from build123d import *

# Parameters (mm, degrees)
CUT_EXTRUDE1_START     = -5
CUT_EXTRUDE1_OUTLINE_W = 4.8
CUT_EXTRUDE1_OUTLINE_H = 50
CUT_EXTRUDE1_DEPTH     = 5
BOSS_EXTRUDE1_START    = -5
BOSS_EXTRUDE1_DEPTH    = 5
BOSS_EXTRUDE2_START    = -5
BOSS_EXTRUDE2_DEPTH    = 5
CUT_EXTRUDE2_DEPTH     = 10
BOSS_EXTRUDE3_START    = -5
BOSS_EXTRUDE3_DEPTH    = 5
BOSS_EXTRUDE4_START    = -5
BOSS_EXTRUDE4_DEPTH    = 5


with BuildPart() as part:
    # Cut-Extrude1: read off the stored shape, not the designer's step
    # Cut-Extrude1 outline → Cut-Extrude1 (new body)
    with BuildSketch(Plane.ZY.offset(CUT_EXTRUDE1_START)):
        with BuildLine():
            Line((22, -25), (47, -50))
            Line((47, -50), (115, -50))
            Line((115, -50), (115, 50))
            Line((115, 50), (-115, 50))
            Line((-115, 50), (-115, -50))
            Line((-115, -50), (-47, -50))
            Line((-47, -50), (-22, -25))
            Line((-22, -25), (-22, 0))
            ThreePointArc((-22, 0), (-16.382917933, 14.683323874), (-2.4, 21.868699093))
            Line((-2.4, 21.868699093), (-2.4, 25))
            Line((-2.4, 25), (2.4, 25))
            Line((2.4, 25), (2.4, 21.868699093))
            ThreePointArc((2.4, 21.868699093), (16.382917933, 14.683323874), (22, 0))
            Line((22, 0), (22, -25))
        make_face()
        with BuildLine():
            ThreePointArc((-33.2, -22.75), (-30.95, -25), (-33.2, -27.25))
            Line((-33.2, -27.25), (-93.2, -27.25))
            ThreePointArc((-93.2, -27.25), (-95.45, -25), (-93.2, -22.75))
            Line((-93.2, -22.75), (-33.2, -22.75))
        make_face(mode=Mode.SUBTRACT)
        with BuildLine():
            ThreePointArc((33.2, -27.25), (30.95, -25), (33.2, -22.75))
            Line((33.2, -22.75), (93.2, -22.75))
            ThreePointArc((93.2, -22.75), (95.45, -25), (93.2, -27.25))
            Line((93.2, -27.25), (33.2, -27.25))
        make_face(mode=Mode.SUBTRACT)
        with Locations((-100, 0)):
            Rectangle(CUT_EXTRUDE1_OUTLINE_W, CUT_EXTRUDE1_OUTLINE_H, mode=Mode.SUBTRACT)
        with BuildLine():
            ThreePointArc((-58.2, 19.5), (-38.7, 0), (-58.2, -19.5))
            Line((-58.2, -19.5), (-68.2, -19.5))
            ThreePointArc((-68.2, -19.5), (-87.7, 0), (-68.2, 19.5))
            Line((-68.2, 19.5), (-58.2, 19.5))
        make_face(mode=Mode.SUBTRACT)
        with BuildLine():
            ThreePointArc((-33.2, 27.25), (-30.95, 25), (-33.2, 22.75))
            Line((-33.2, 22.75), (-93.2, 22.75))
            ThreePointArc((-93.2, 22.75), (-95.45, 25), (-93.2, 27.25))
            Line((-93.2, 27.25), (-33.2, 27.25))
        make_face(mode=Mode.SUBTRACT)
        with BuildLine():
            ThreePointArc((58.2, -19.5), (38.7, 0), (58.2, 19.5))
            Line((58.2, 19.5), (68.2, 19.5))
            ThreePointArc((68.2, 19.5), (87.7, 0), (68.2, -19.5))
            Line((68.2, -19.5), (58.2, -19.5))
        make_face(mode=Mode.SUBTRACT)
        with Locations((100, 0)):
            Rectangle(CUT_EXTRUDE1_OUTLINE_W, CUT_EXTRUDE1_OUTLINE_H, mode=Mode.SUBTRACT)
        with BuildLine():
            ThreePointArc((33.2, 22.75), (30.95, 25), (33.2, 27.25))
            Line((33.2, 27.25), (93.2, 27.25))
            ThreePointArc((93.2, 27.25), (95.45, 25), (93.2, 22.75))
            Line((93.2, 22.75), (33.2, 22.75))
        make_face(mode=Mode.SUBTRACT)
    extrude(amount=CUT_EXTRUDE1_DEPTH)

    # Sketch2 → Boss-Extrude1 (add)
    with BuildSketch(Plane.ZY.offset(BOSS_EXTRUDE1_START)):
        with BuildLine():
            Line((2.4, 25), (-2.4, 25))
            Line((-2.4, 25), (-2.4, 21.868699093))
            ThreePointArc((-2.4, 21.868699093), (0, 22), (2.4, 21.868699093))
            Line((2.4, 21.868699093), (2.4, 25))
        make_face()
    extrude(amount=BOSS_EXTRUDE1_DEPTH)

    # Sketch3 → Boss-Extrude2 (add)
    with BuildSketch(Plane.ZY.offset(BOSS_EXTRUDE2_START)):
        with BuildLine():
            Line((13.5, -50), (13.5, 17.370952766))
            ThreePointArc((13.5, 17.370952766), (0, 22), (-13.5, 17.370952766))
            Line((-13.5, 17.370952766), (-13.5, -50))
            Line((-13.5, -50), (13.5, -50))
        make_face()
    extrude(amount=BOSS_EXTRUDE2_DEPTH)

    # Sketch4 → Cut-Extrude2 (cut)
    with BuildSketch(Plane.ZY):
        with BuildLine():
            Line((7, -18), (7, -50))
            ThreePointArc((7, -50), (0, -57), (-7, -50))
            Line((-7, -50), (-7, -18))
            ThreePointArc((-7, -18), (0, -11), (7, -18))
        make_face()
    extrude(amount=-CUT_EXTRUDE2_DEPTH, mode=Mode.SUBTRACT)

    # Sketch5 → Boss-Extrude3 (add)
    with BuildSketch(Plane.ZY.offset(BOSS_EXTRUDE3_START)):
        Polygon((-22, -25), (-22, -50), (-47, -50), align=None)
        with BuildLine():
            Line((-13.5, 17.370952766), (-13.5, 0))
            ThreePointArc((-13.5, 0), (-17.75, 4.25), (-22, 0))
            ThreePointArc((-22, 0), (-19.761072845, 9.669539803), (-13.5, 17.370952766))
        make_face()
    boss_extrude3 = extrude(amount=BOSS_EXTRUDE3_DEPTH)

    # Sketch6 → Boss-Extrude4 (add)
    with BuildSketch(Plane.ZY.offset(BOSS_EXTRUDE4_START)):
        with BuildLine():
            Line((-13.5, 0), (-13.5, -17))
            ThreePointArc((-13.5, -17), (-17.75, -12.75), (-22, -17))
            Line((-22, -17), (-22, 0))
            ThreePointArc((-22, 0), (-17.75, 4.25), (-13.5, 0))
        make_face()
    boss_extrude4 = extrude(amount=BOSS_EXTRUDE4_DEPTH)

    # Mirror1: Boss-Extrude3, Boss-Extrude4 across plane
    add(boss_extrude3.mirror(Plane.XY))
    add(boss_extrude4.mirror(Plane.XY))


solid = part.part
For this review, take the finished solid that the model builds, in its own axes (mm). A direction names the side the tool comes from. Coordinates: 2 decimals unless noted, no trailing zeros. Order: outer loops, then holes, each group sorted by start corner. A loop starts at its lowest first (then second) coordinate and runs counter-clockwise, first axis right, second up. Notation, with made-up numbers: (-26.75, 21) - (-22.75, 21) arc R11 ccw to (-22.75, 40) - close; hole circle Ø10 at (-10.75, -23.75). An arc over 180 degrees is marked (long way). Use one line per item in the form item = value.
Q1. Consider section A-A (y = -35). Give the boundary of the cut face in (x, z).
Checked values:
outline = (0, -115) - (5, -115) - (5, -22) - (0, -22) - close; (0, -13.5) - (5, -13.5) - (5, -7) - (0, -7) - close; (0, 7) - (5, 7) - (5, 13.5) - (0, 13.5) - close; (0, 22) - (5, 22) - (5, 115) - (0, 115) - close
Q2. For probe 1 along Y at (x, z) = (3, 36.5); probe 2 along Y at (x, z) = (1.35, 62); probe 3 along Z at (x, y) = (2.1, -39.5), list the stretches that pass through material, from the lowest coordinate up. Write a range as from..to.
Checked values:
probe_1 = -50..-27.25, -22.75..22.75, 27.25..50
probe_2 = -50..-27.25, -22.75..-19.5, 19.5..22.75, 27.25..50
probe_3 = -115..-22, -13.5..-7, 7..13.5, 22..115
Q3. Draft analysis for pull direction Z (two halves, no side actions). For faces 1 (the flat face through (3, -50, -68)), 2 (the flat face through (3, 25, 100)), state which applies: +Z half, -Z half, draft (parallel to the pull), parting line (faces both ways), or undercut.
Checked values:
face_1 = draft
face_2 = undercut
Q4. Consider section D-D (x = 1). Give the number of separate pieces and of enclosed holes in the cut face, then the cut area to 3 significant figures.
Checked values:
separate_pieces = 1
enclosed_holes = 8
area = 17,100 mm2
Q5. Consider section C-C (z = -76.5). Give the boundary of the cut face in (x, y).
Checked values:
outline = (0, -50) - (5, -50) - (5, -27.25) - (0, -27.25) - close; (0, -22.75) - (5, -22.75) - (5, -17.65) - (0, -17.65) - close; (0, 17.65) - (5, 17.65) - (5, 22.75) - (0, 22.75) - close; (0, 27.25) - (5, 27.25) - (5, 50) - (0, 50) - close
Q6. For faces 3 (the flat face through (2, -34, -7)), 4 (the flat face through (0, 1, -2)), 5 (the flat face through (3, 19.5, 63)), list the 3-axis set-ups (+Z, -Z, +X, -X, +Y, -Y) from which the entire face can be reached by the end or side of a thin tool; tool diameter is ignored.
Checked values:
face_3 = +X, -X, -Y
face_4 = +Z, -Z, -X, +Y, -Y
face_5 = +X, -X
Q7. Consider section B-B (y = 0). Give the boundary of the cut face in (x, z).
Checked values:
outline = (0, -115) - (5, -115) - (5, -102.4) - (0, -102.4) - close; (0, -97.6) - (5, -97.6) - (5, -87.7) - (0, -87.7) - close; (0, -38.7) - (5, -38.7) - (5, 38.7) - (0, 38.7) - close; (0, 87.7) - (5, 87.7) - (5, 97.6) - (0, 97.6) - close; (0, 102.4) - (5, 102.4) - (5, 115) - (0, 115) - close
